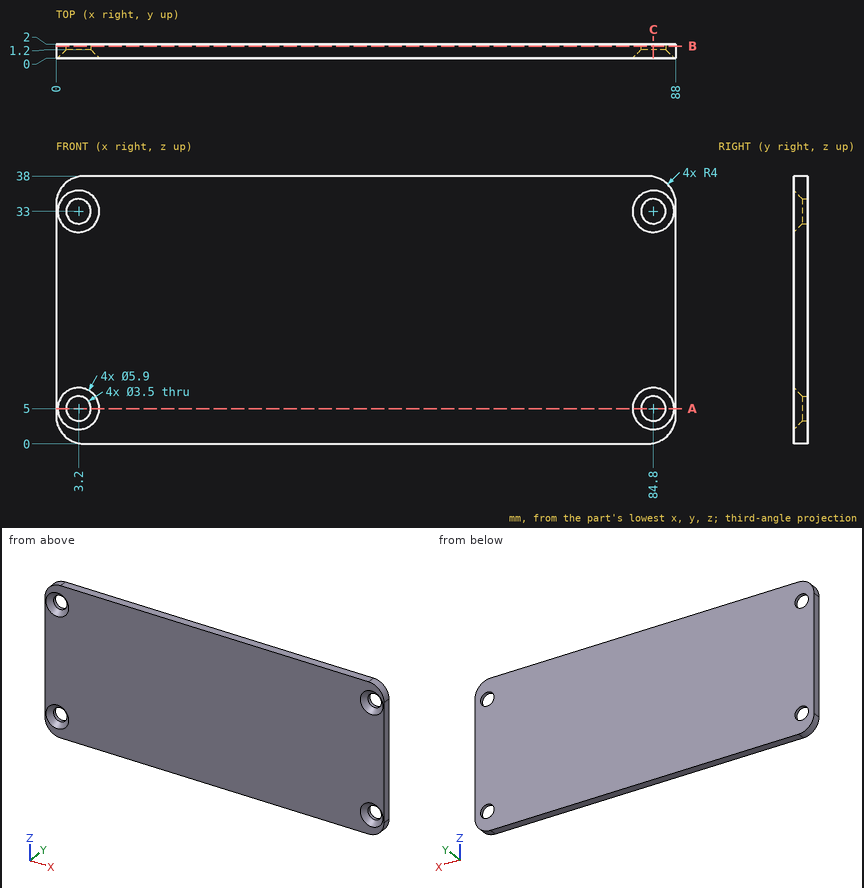
Could you check a few things on this drawing? It's one solid part, dimensions in mm from its lowest x, y, z. Give positions to 0.01 mm unless a question says otherwise; leave off trailing zeros. Write each loop counter-clockwise with the first axis right and the second up, starting at its lowest first coordinate (ties: lowest second). Pieces come first, ordered by that corner, then holes. Notation, with made-up numbers: (48, 30) -> (95, 30) arc R21 cw to (95, 65) -> close; hole circle Ø5 at (17.25, 18). An arc over 180 degrees is marked (long way). Answer as a JSON object with one key per item and string values.
Q1. Please list where these lines run through material, in increasing order: L1, parallel to Z at x = 84.8, y = 1.45; L2, parallel to X at y = 1.1, z = 5.5; L3, parallel to X at y = 1.15, z = 6.5.
Taken from the geometry:
{"L1": "z = 0.08 to 3.25, 6.75 to 31.25, 34.75 to 37.92", "L2": "x = 0 to 1.42, 4.98 to 83.02, 86.58 to 88", "L3": "x = 0 to 2.21, 4.19 to 83.81, 85.79 to 88"}
Q2. Suppose I cut it at A-A on z = 5. Write out the boundary of the cut face in (x, y).
Taken from the geometry:
{"outline": "(0, 0) -> (0.25, 0) -> (1.45, 1.2) -> (1.45, 2) -> (0, 2) -> close; (4.95, 1.2) -> (6.15, 0) -> (81.85, 0) -> (83.05, 1.2) -> (83.05, 2) -> (4.95, 2) -> close; (86.55, 1.2) -> (87.75, 0) -> (88, 0) -> (88, 2) -> (86.55, 2) -> close"}
Q3. Will these pins go through, and if not, where does the flat tip stop? pin 1 Ø2 at (x, z) = (3.2, 5) entering from -Y; pin 2 Ø5.5 at (x, z) = (3.2, 33) entering from -Y.
Taken from the geometry:
{"pin 1": "passes through", "pin 2": "stops at y = 0.2"}
Q4. Suppose I cut it at C-C on x = 84.8. Write out the boundary of the cut face in (y, z).
Taken from the geometry:
{"outline": "(0, 0.08) -> (2, 0.08) -> (2, 3.25) -> (1.2, 3.25) -> (0, 2.05) -> close; (0, 7.95) -> (1.2, 6.75) -> (2, 6.75) -> (2, 31.25) -> (1.2, 31.25) -> (0, 30.05) -> close; (0, 35.95) -> (1.2, 34.75) -> (2, 34.75) -> (2, 37.92) -> (0, 37.92) -> close"}
Q5. Suppose I cut it at B-B on y = 1.7. Write out the boundary of the cut face in (x, z).
Taken from the geometry:
{"outline": "(0, 4) arc R4 ccw to (4, 0) -> (84, 0) arc R4 ccw to (88, 4) -> (88, 34) arc R4 ccw to (84, 38) -> (4, 38) arc R4 ccw to (0, 34) -> close; hole circle Ø3.5 at (3.2, 5); hole circle Ø3.5 at (3.2, 33); hole circle Ø3.5 at (84.8, 5); hole circle Ø3.5 at (84.8, 33)"}
